Source: CAD feature listing. Evaluate the final solid. Frame: model axes, mm. Face numbers are marked on the shaded views. Coordinates: 2 decimals unless noted, no trailing zeros. Order: outer loops, then holes, each group sorted by start corner. A loop starts at its lowest first (then second) coordinate and runs counter-clockwise, first axis right, second up.
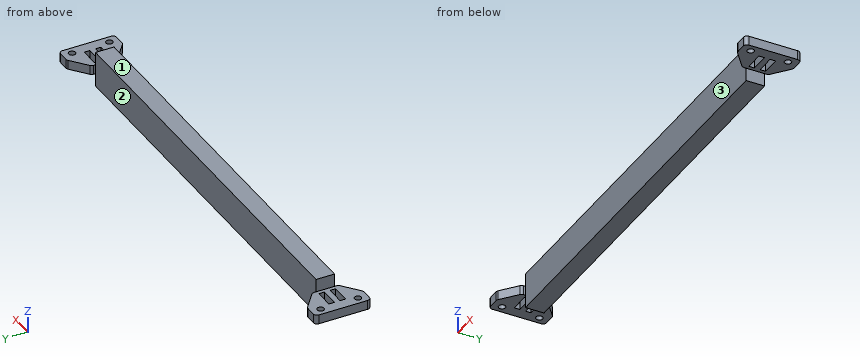
```python
from build123d import *

# Parameters (mm, degrees)
SKETCH1_R           = 2.286
SKETCH1_W           = 12.7
SKETCH1_H           = 3.81
BOSS_EXTRUDE1_DEPTH = 3.175
FILLET1_R           = 2.54
SKETCH3_W           = 279.4
SKETCH3_H           = 12.573
BOSS_EXTRUDE3_DEPTH = 8.89


with BuildPart() as part:
    # Sketch1 → Boss-Extrude1 (new, symmetric)
    with BuildSketch(Plane.XY):
        Polygon((-139.7, -6.2865), (139.7, -6.2865), (139.7, -8.8265), (152.4, -19.05), (162.56, -19.05), (162.56, 19.05), (152.4, 19.05), (139.7, 8.8265), (139.7, 6.2865), (-139.7, 6.2865), (-139.7, 8.8265), (-152.4, 19.05), (-162.56, 19.05), (-162.56, -19.05), (-152.4, -19.05), (-139.7, -8.8265), align=None)
        with Locations((-157.48, -12.7)):
            Circle(SKETCH1_R, mode=Mode.SUBTRACT)
        with Locations(Location((-157.48, 12.7, 0), (0, 0, 180))):
            Circle(SKETCH1_R, mode=Mode.SUBTRACT)
        with Locations((157.48, 12.7)):
            Circle(SKETCH1_R, mode=Mode.SUBTRACT)
        with Locations(Location((157.48, -12.7, 0), (0, 0, 180))):
            Circle(SKETCH1_R, mode=Mode.SUBTRACT)
        with Locations((-148.59, 3.81)):
            Rectangle(SKETCH1_W, SKETCH1_H, mode=Mode.SUBTRACT)
        with Locations((-148.59, -3.81)):
            Rectangle(SKETCH1_W, SKETCH1_H, mode=Mode.SUBTRACT)
        with Locations((148.59, -3.81)):
            Rectangle(SKETCH1_W, SKETCH1_H, mode=Mode.SUBTRACT)
        with Locations((148.59, 3.81)):
            Rectangle(SKETCH1_W, SKETCH1_H, mode=Mode.SUBTRACT)
    extrude(amount=BOSS_EXTRUDE1_DEPTH, both=True)

    # Fillet1
    fillet1_edges = [part.edges().sort_by_distance(p)[0] for p in [
        (-139.7, -8.8265, 0),
        (-152.4, -19.05, 0),
        (-162.56, -19.05, 0),
        (-162.56, 19.05, 0),
        (-152.4, 19.05, 0),
        (-139.7, 8.8265, 0),
        (139.7, 8.8265, 0),
        (152.4, 19.05, 0),
        (162.56, 19.05, 0),
        (162.56, -19.05, 0),
        (152.4, -19.05, 0),
        (139.7, -8.8265, 0),
    ]]
    fillet(fillet1_edges, radius=FILLET1_R)

    # Sketch3 → Boss-Extrude3 (add)
    with BuildSketch(Plane.XY.offset(3.175)):
        Rectangle(SKETCH3_W, SKETCH3_H)
    boss_extrude3 = extrude(amount=BOSS_EXTRUDE3_DEPTH)

    # Mirror1: Boss-Extrude3 across plane
    add(boss_extrude3.mirror(Plane.XY))


solid = part.part
```
1. Section query B-B on x = -85. Return loops of the section in (y, z) (1 decimal).
Findings:
outline: (-6.3, -12.1) - (6.3, -12.1) - (6.3, 12.1) - (-6.3, 12.1) - close
2. Section query A-A on z = 9.25. Return loops of the section in (x, y), plus the area to 3 significant figures.
Findings:
outline: (-139.7, -6.29) - (139.7, -6.29) - (139.7, 6.29) - (-139.7, 6.29) - close
area: 3,510 mm2
3. Ray query, line 1 (Y direction, x = 157.48, z = 0.5); line 2 (X direction, y = -11.5, z = 3); line 3 (X direction, y = -13.5, z = 2.5). Return the intervals inside material, ascending.
Findings:
line 1: y = -19.05 to -14.99, -10.41 to 10.41, 14.99 to 19.05
line 2: x = -162.56 to -159.43, -155.53 to -143.02, 143.02 to 155.53, 159.43 to 162.56
line 3: x = -162.56 to -159.62, -155.34 to -145.51, 145.51 to 155.34, 159.62 to 162.56
4. Draft query along X for the marked faces 1, 2 and 3. Return one class per face: released by +X, released by -X, zero draft, split by the parting line, or undercut.
Findings:
face 1: zero draft
face 2: undercut
face 3: undercut
5. Pin query (flat end, axial travel): P1, Ø1.9, axis at x = -147, z = -1, coming from the -Y side; P2, Ø1.9, axis at x = 150.5, z = 0, coming from the +Y side; P3, Ø1, axis at x = -72.5, z = -0.5, coming from the -Y side. Return the tip coordinate at first contact, or that it passes through.
Findings:
P1: stops at y = -15.47
P2: stops at y = 18.29
P3: stops at y = -6.29
